Verification items for this drawing (mm, ordinates from the low corner). A direction names the side the tool comes from. Coordinates: 2 decimals unless noted, no trailing zeros. Loops run counter-clockwise (first coordinate to the right, second up) from the corner with the lowest first, then second, coordinate; pieces in that order, holes last.
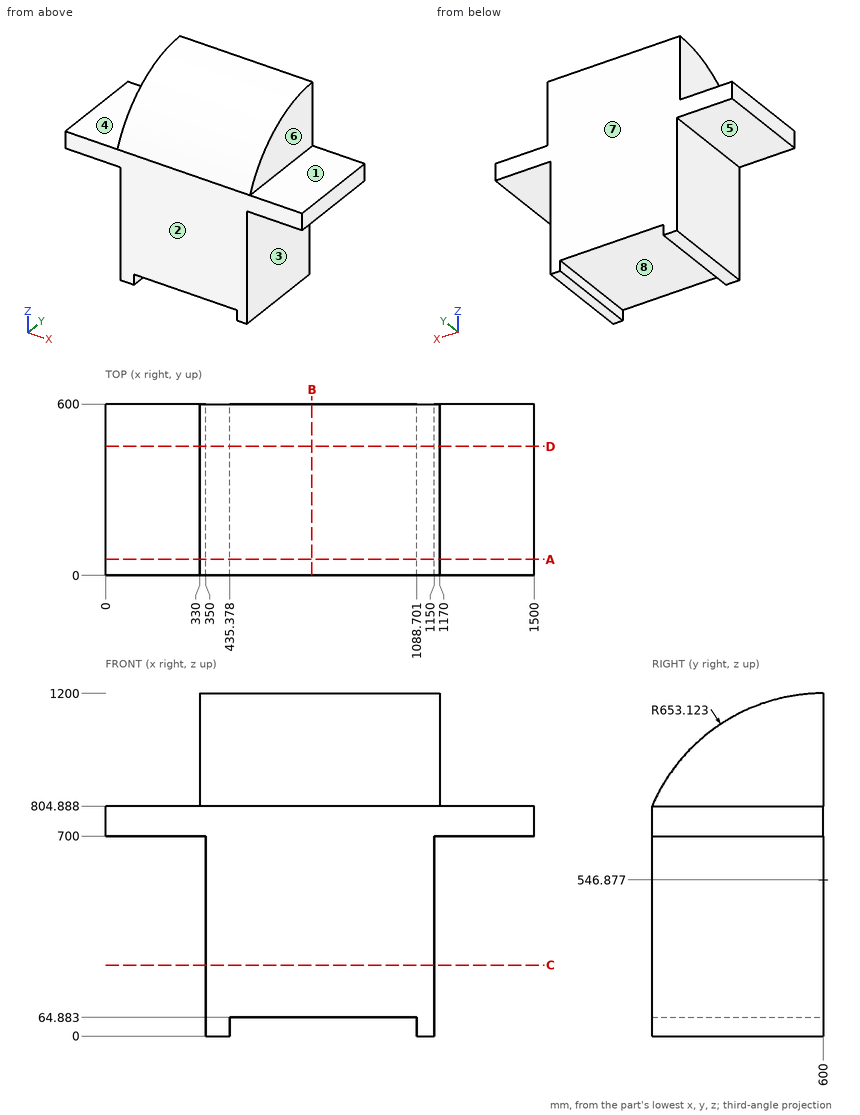
(1) Scan lines: line 1 along X through (y, z) = (179, 53); line 2 along X through (y, z) = (185.5, 651); line 3 along Z through (x, y) = (110.5, 477). Record each from-to range of solid material in increasing order.
(2) Draft check along X on the marked faces 6, 7 and 8. Enter one of: pulls with the +X half, pulls with the -X half, needs draft (parallel to the pull), parting line crosses it, or undercut.
(3) Gauge pin test, flat ends, axial feed: P1, Ø2, axis at y = 171, z = 241, coming from the -X side; P2, Ø4, axis at y = 229, z = 1033, coming from the +X side; P3, Ø10, axis at y = 249.5, z = 1033, coming from the -X side. Record the tip position at first contact, or that the pin passes through.
(4) Set-up check for the marked faces 1, 2, 3, 4 and 5: record each of +Z, -Z, +X, -X, +Y, -Y from which the full face is reachable in a straight line by a thin tool's end or side.
(5) Section check B-B, the plane x = 722. Enter the section's corners in (y, z) (1 decimal).
(6) Section check C-C, the plane z = 248. Enter the section's corners in (x, y).
(7) Section check D-D, the plane y = 451.5. Enter the section's corners in (x, z).
(8) Section check A-A, the plane y = 55.5. Enter the section's corners in (x, z), plus the area to 3 significant figures.
Determined:
1. line 1: x = 350 to 435.38, 1088.7 to 1150
1. line 2: x = 350 to 1150
1. line 3: z = 700 to 804.89
2. face 6: pulls with the +X half
2. face 7: needs draft
2. face 8: undercut
3. P1: stops at x = 350
3. P2: stops at x = 1170
3. P3: stops at x = 330
4. face 1: +Z, +X, +Y, -Y
4. face 2: +Z, -Z, +X, -X, -Y
4. face 3: -Z, +X, +Y, -Y
4. face 4: +Z, -X, +Y, -Y
4. face 5: -Z, -X, +Y, -Y
5. outline: (0, 64.9) - (600, 64.9) - (600, 1200) arc R653.1 ccw to (0, 804.9) - close
6. outline: (350, 0) - (1150, 0) - (1150, 600) - (350, 600) - close
7. outline: (0, 700) - (350, 700) - (350, 0) - (435.38, 0) - (435.38, 64.88) - (1088.7, 64.88) - (1088.7, 0) - (1150, 0) - (1150, 700) - (1500, 700) - (1500, 804.89) - (1170, 804.89) - (1170, 1182.89) - (330, 1182.89) - (330, 804.89) - (0, 804.89) - close
8. outline: (0, 700) - (350, 700) - (350, 0) - (435.38, 0) - (435.38, 64.88) - (1088.7, 64.88) - (1088.7, 0) - (1150, 0) - (1150, 700) - (1500, 700) - (1500, 804.89) - (1170, 804.89) - (1170, 907.56) - (330, 907.56) - (330, 804.89) - (0, 804.89) - close
8. area: 761,000 mm2
